```python
from build123d import *

# Parameters (mm, degrees)
F1_DEPTH = 1
F2_R     = 2.5
F3_DEPTH = 4
F4_R     = 1
F5_DEPTH = 25


with BuildPart() as f1:
    # F0 (on Top) → F1 (new body)
    with BuildSketch(Plane.XY):
        Polygon((21.213203, 0), (0, 21.213203), (-21.213203, 0), (0, -21.213203), align=None)
    extrude(amount=F1_DEPTH)

    # F2 (on face) → F3 (join)
    with BuildSketch(Plane.XY.offset(1)):
        with Locations((-15, 0)):
            Circle(F2_R)
        with Locations((15, 0)):
            Circle(F2_R)
    extrude(amount=F3_DEPTH)

    # F4 (on face) → F5 (cut)
    with BuildSketch(Plane.XY.offset(5)):
        with Locations((-15, 0)):
            Circle(F4_R)
        with Locations((15, 0)):
            Circle(F4_R)
    extrude(amount=-F5_DEPTH, mode=Mode.SUBTRACT)


solid = f1.part
```
Could you check a few things on this model? Use its own coordinates, in mm. A direction names the side the tool comes from. Round coordinates to 2 decimals unless told otherwise and drop trailing zeros. Loops run counter-clockwise (first coordinate to the right, second up) from the corner with the lowest first, then second, coordinate; pieces in that order, holes last. Notation, with made-up numbers: (51, 78.25) - (61, 78.25) arc R25 cw to (61, 113.25) - close; hole circle Ø9 at (70.25, -33). An arc over 180 degrees is marked (long way). Use CSV: the item, a comma, the result in double quotes.
Item 1: If we section it at D-D on x = 10: List the corners of the cut face in (y, z) for me, then the cut area to 3 significant figures.
Here are the results:
outline,"(-11.21, 0) - (11.21, 0) - (11.21, 1) - (-11.21, 1) - close"
area,"22.4 mm²"
Item 2: For faces 5 (the cylindrical face through (12.5, 0.1, 3)), 6 (the flat face through (-10.755, -10.458, 0.493)), which set-ups out of +Z, -Z, +X, -X, +Y, -Y let a thin tool reach every point of the face, with its end or its side?
Here are the results:
face 5,"+Z"
face 6,"+Z, -Z, -X, -Y"
Item 3: Will these pins go through, and if not, where does the flat tip stop? pin 1 (3 mm diameter, centred on x = 9, z = 1, fed in from +Y); pin 2 (1 mm diameter, centred on x = -6, z = 1, fed in from +Y).
Here are the results:
pin 1,"stops at y = 13.71"
pin 2,"stops at y = 15.71"
Item 4: If we section it at C-C on y = -18: List the corners of the cut face in (x, z) for me, then the cut area to 3 significant figures.
Here are the results:
outline,"(-3.21, 0) - (3.21, 0) - (3.21, 1) - (-3.21, 1) - close"
area,"6.43 mm²"
Item 5: If we section it at A-A on z = 3.2: List the corners of the cut face in (x, y) for me.
Here are the results:
outline,"circle Ø5 at (-15, 0); circle Ø5 at (15, 0); hole circle Ø2 at (-15, 0); hole circle Ø2 at (15, 0)"
Item 6: I need wall thicknesses on L1, parallel to Y at x = -15, z = 2.35; L2, parallel to Z at x = 13, y = -2; L3, parallel to X at y = 2, z = 3.5. Which ranges of each line are inside material? Lowest first, please. Write a range as [from, to].
Here are the results:
L1,"y = [-2.5, -1], [1, 2.5]"
L2,"z = [0, 1]"
L3,"x = [-16.5, -13.5], [13.5, 16.5]"
Item 7: If we mould it in two halves opening along Y, with no side actions, what happens to faces 1 (the cylindrical face through (-14, 0, 3)), 2 (the cylindrical face through (16, 0, 3)), 3 (the flat face through (-14, -1, 5)), 4 (the flat face through (10.755, 10.458, 0.493))? For each: pulls with the +Y half, pulls with the -Y half, needs draft (parallel to the pull), parting line crosses it, or undercut.
Here are the results:
face 1,"undercut"
face 2,"undercut"
face 3,"needs draft"
face 4,"pulls with the +Y half"
Item 8: If we section it at B-B on x = -14.5: List the corners of the cut face in (y, z) for me.
Here are the results:
outline,"(-6.71, 0) - (-0.87, 0) - (-0.87, 5) - (-2.45, 5) - (-2.45, 1) - (-6.71, 1) - close; (0.87, 0) - (6.71, 0) - (6.71, 1) - (2.45, 1) - (2.45, 5) - (0.87, 5) - close"
